Geometry: final body of the model. Coordinates: model frame, mm. A direction names the side the tool comes from. Give positions to 0.01 mm unless a question says otherwise; leave off trailing zeros. Loops run counter-clockwise (first coordinate to the right, second up) from the corner with the lowest first, then second, coordinate; pieces in that order, holes last.
1. Section C-C, the plane z = -17.78. Output: boundary loops of the cut face in (x, y), then the cut area to 3 significant figures.
2. First-contact query: P1, Ø10, axis at x = 13, z = -44.5, coming from the -Y side; P2, Ø8.5, axis at x = 6, y = 5.5, coming from the +Z side; P3, Ø10, axis at x = 13, y = 12.5, coming from the -Z side; P4, Ø2, axis at y = 16.5, z = -28.5, coming from the -X side. Flat tips, straight axial feed; report the tip coordinate or a pass-through.
3. Material intervals for line 1 along Y through (x, z) = (12.7, -32.75); line 2 along Y through (x, z) = (2, -6); line 3 along X through (y, z) = (22, -33), sorted ascending.
4. Section A-A, the plane y = 22.86. Output: boundary loops of the cut face in (x, z), then the cut area to 3 significant figures.
5. Access query for faces 1 (the face through (12.7, 35, -48)), 2 (the face through (6, 4, -12.7)), 3 (the face through (10, 31.707, -43)), 4 (the face through (23.56, 11.38, -20.12)), 5 (the face through (19, 15.24, -18)). Directions: +Z, -Z, +X, -X, +Y, -Y. A direction counts if a zero-diameter tool reaches every point of the face in a straight line with its end or side. Return the directions, or none.
6. Section B-B, the plane x = 2.5. Output: boundary loops of the cut face in (y, z), then the cut area to 3 significant figures.
7. Section D-D, the plane x = 10.25. Output: boundary loops of the cut face in (y, z).
8. Draft query along Z for faces 6 (the face through (19, 35, -44.45)), 7 (the face through (25.4, 15, -32)), 8 (the face through (13, 7.62, -12)). Return one class per face: +Z half, -Z half, draft (parallel to the pull), parting line (faces both ways), or undercut.
from build123d import *

# Parameters (mm, degrees)
SKETCH1_W               = 25.4
SKETCH1_H               = 50.8
BOSS_EXTRUDE1_DEPTH     = 38.1
SKETCH2_W               = 25.4
SKETCH2_H               = 30.48
CUT_EXTRUDE1_DEPTH      = 30.48
CUT_EXTRUDE2_DEPTH      = 10.668
CUT_EXTRUDE2_DEPTH_BACK = 32.258
SKETCH3_W               = 12.7
SKETCH3_H               = 31.706835607
SKETCH4_W               = 12.7
SKETCH4_H               = 6.35
CUT_EXTRUDE3_DEPTH      = 32.258
CHAMFER1_SIZE           = 6.35
FILLET1_R               = 12.7
FILLET2_R               = 12.7
SKETCH8_R               = 5.08
BOSS_EXTRUDE3_DEPTH     = 7.62
SKETCH9_R               = 6.35
CUT_EXTRUDE6_DEPTH      = 7.62
SKETCH10_W              = 12.7
SKETCH10_H              = 12.7
CUT_EXTRUDE7_DEPTH      = 7.62


with BuildPart() as part:
    # Sketch1 → Boss-Extrude1 (new body)
    with BuildSketch(Plane(origin=(0, 0, 0), x_dir=(1, 0, 0), z_dir=(0, 1, 0))):
        with Locations((12.7, 25.4)):
            Rectangle(SKETCH1_W, SKETCH1_H)
    extrude(amount=BOSS_EXTRUDE1_DEPTH)

    # Sketch2 → Cut-Extrude1 (cut)
    with BuildSketch(Plane(origin=(0, 38.1, 0), x_dir=(1, 0, 0), z_dir=(0, 1, 0))):
        with Locations((12.7, 15.24)):
            Rectangle(SKETCH2_W, SKETCH2_H)
    extrude(amount=-CUT_EXTRUDE1_DEPTH, mode=Mode.SUBTRACT)

    # Sketch3 → Cut-Extrude2 (cut, two sides: drawn at the far end of the back side and taken through both)
    with BuildSketch(Plane.ZY.offset(-CUT_EXTRUDE2_DEPTH_BACK)):
        with Locations((-44.45, 15.853417804)):
            Rectangle(SKETCH3_W, SKETCH3_H)
    extrude(amount=CUT_EXTRUDE2_DEPTH + CUT_EXTRUDE2_DEPTH_BACK, mode=Mode.SUBTRACT)

    # Sketch4 → Cut-Extrude3 (cut)
    with BuildSketch(Plane(origin=(0, 38.1, 0), x_dir=(1, 0, 0), z_dir=(0, 1, 0))):
        with Locations((19.05, 47.625)):
            Rectangle(SKETCH4_W, SKETCH4_H)
    extrude(amount=-CUT_EXTRUDE3_DEPTH, mode=Mode.SUBTRACT)

    # Chamfer1
    chamfer1_edges = [part.edges().sort_by_distance(p)[0] for p in [
        (0, 34.903417804, -50.8),
    ]]
    chamfer(chamfer1_edges, length=CHAMFER1_SIZE)

    # Fillet1
    fillet1_edges = [part.edges().sort_by_distance(p)[0] for p in [
        (25.4, 3.81, 0),
    ]]
    fillet(fillet1_edges, radius=FILLET1_R)

    # Fillet2
    fillet2_edges = [part.edges().sort_by_distance(p)[0] for p in [
        (0, 3.81, 0),
    ]]
    fillet(fillet2_edges, radius=FILLET2_R - 0.0001)  # a hair under: the kernel refuses the full size

    # Sketch8 → Boss-Extrude3 (add)
    with BuildSketch(Plane(origin=(0, 7.62, 0), x_dir=(1, 0, 0), z_dir=(0, 1, 0))):
        with Locations(Location((19.05, 17.78, 0), (0, 0, 90))):
            Circle(SKETCH8_R)
    extrude(amount=BOSS_EXTRUDE3_DEPTH)

    # Sketch9 → Cut-Extrude6 (cut)
    with BuildSketch(Plane.XY.offset(-30.48)):
        with Locations((12.7, 22.86)):
            Circle(SKETCH9_R)
    extrude(amount=-CUT_EXTRUDE6_DEPTH, mode=Mode.SUBTRACT)

    # Sketch10 → Cut-Extrude7 (cut)
    with BuildSketch(Plane(origin=(0, 7.62, 0), x_dir=(1, 0, 0), z_dir=(0, 1, 0))):
        with Locations((6.35, 19.05)):
            Rectangle(SKETCH10_W, SKETCH10_H)
    extrude(amount=-CUT_EXTRUDE7_DEPTH, mode=Mode.SUBTRACT)


solid = part.part
Answers below:
1. outline: (12.7, 0) - (25.4, 0) - (25.4, 7.62) - (24.13, 7.62) - (24.13, 15.24) - (13.97, 15.24) - (13.97, 7.62) - (12.7, 7.62) - close
1. area: 174 mm2
2. P1: stops at y = 31.71
2. P2: stops at z = -0.24
2. P3: stops at z = -38.1
2. P4: passes through
3. line 1: y = 0 to 16.51, 29.21 to 38.1
3. line 2: y = 0 to 7.62
3. line 3: x = 0 to 6.41, 18.99 to 25.4
4. outline: (0, -38.1) - (6.35, -38.1) - (6.35, -30.48) - (0, -30.48) - close; (19.05, -38.1) - (25.4, -38.1) - (25.4, -30.48) - (19.05, -30.48) - close
4. area: 96.8 mm2
5. face 1: -Z, +X, +Y, -Y
5. face 2: -X, +Y, -Y
5. face 3: -Z, +X, -X, -Y
5. face 4: +Y
5. face 5: +Z, +X, -X, +Y
6. outline: (0, -38.1) - (31.71, -38.1) - (31.71, -46.95) - (38.1, -46.95) - (38.1, -30.48) - (7.62, -30.48) - (7.62, -25.4) - (0, -25.4) - close; (0, -12.7) - (7.62, -12.7) - (7.62, -5.13) - (0, -5.13) - close
6. area: 443 mm2
7. outline: (0, -38.1) - (17, -38.1) - (17, -30.48) - (7.62, -30.48) - (7.62, -25.4) - (0, -25.4) - close; (0, -12.7) - (7.62, -12.7) - (7.62, -0.24) - (0, -0.24) - close; (28.72, -38.1) - (31.71, -38.1) - (31.71, -50.8) - (38.1, -50.8) - (38.1, -30.48) - (28.72, -30.48) - close
8. face 6: -Z half
8. face 7: draft
8. face 8: undercut
